from build123d import *

# Parameters (mm, degrees)
SKETCH1_R                       = 4.7625
BOSS_EXTRUDE1_DEPTH             = 6.35
F_14_0_182_DIAMETER_HOLE1_D     = 4.6228
F_14_0_182_DIAMETER_HOLE1_DEPTH = 2.54
F_14_0_182_DIAMETER_HOLE1_TIP   = 1.388829235


with BuildPart() as part:
    # Sketch1 → Boss-Extrude1 (new body)
    with BuildSketch(Plane(origin=(0, 0, 0), x_dir=(1, 0, 0), z_dir=(0, 1, 0))):
        with BuildLine():
            Line((-2.715472603, -50.452570894), (-16.449210706, -36.716165316))
            Line((-16.449210706, -36.716165316), (-7.143929399, -5.302062091))
            ThreePointArc((-7.143929399, -5.302062091), (-4.881213446, -3.126502672), (-1.85461271, -3.95874678))
            Line((-1.85461271, -3.95874678), (13.315573809, -19.128933299))
            Line((13.315573809, -19.128933299), (15.879471691, -10.753687697))
            Line((15.879471691, -10.753687697), (2.2197595, 40.561165667))
            Line((2.2197595, 40.561165667), (-6.994225827, 38.108456959))
            Line((-6.994225827, 38.108456959), (-46.728023778, -55.399752843))
            Line((-46.728023778, -55.399752843), (-12.38156047, -66.157106701))
            ThreePointArc((-12.38156047, -66.157106701), (-1.47172138, -62.045085351), (-2.715472603, -50.452570894))
        make_face()
        with Locations(Location((-9.583361485, -57.052398719, 0), (0, 0, 270))):
            Circle(SKETCH1_R, mode=Mode.SUBTRACT)
    extrude(amount=BOSS_EXTRUDE1_DEPTH)

    # #14 (0.182) Diameter Hole1
    with Locations(Plane(origin=(-19.975553156, 0, 63.778659005), x_dir=(0.9542892760421928, 0, 0.29888455569143674), z_dir=(-0.29888455569143674, 0, 0.9542892760421928))):
        with Locations((-25.620921468, 3.175)):
            Hole(F_14_0_182_DIAMETER_HOLE1_D / 2, depth=F_14_0_182_DIAMETER_HOLE1_DEPTH)
            with Locations((0, 0, -(F_14_0_182_DIAMETER_HOLE1_DEPTH + F_14_0_182_DIAMETER_HOLE1_TIP / 2))):  # 118° drill point
                Cone(0, F_14_0_182_DIAMETER_HOLE1_D / 2, F_14_0_182_DIAMETER_HOLE1_TIP, mode=Mode.SUBTRACT)


solid = part.part
Could you check a few things on this model? Use its own coordinates, in mm. A direction names the side the tool comes from. Coordinates: 2 decimals unless noted, no trailing zeros. Write each loop counter-clockwise with the first axis right and the second up, starting at its lowest first coordinate (ties: lowest second). Pieces come first, ordered by that corner, then holes. Notation, with made-up numbers: (19.25, -39.5) - (68.25, -39.5) arc R31 cw to (68.25, -9.5) - close; hole circle Ø5 at (-4, 79). An arc over 180 degrees is marked (long way). Write item = value, one per line.
1) Suppose I cut it at A-A on z = 7. Please give me the cut outline in (x, y).
Result set:
outline = (-26.16, 0) - (-7.65, 0) - (-7.65, 6.35) - (-26.16, 6.35) - close; (1.19, 0) - (14.88, 0) - (14.88, 6.35) - (1.19, 6.35) - close
2) For faces 1 (the flat face through (-9.486, 3.131, 43.681)), 2 (the cylindrical face through (-4.93, 3.13, 3.14)), 3 (the flat face through (-26.583, 3.131, 7.991)), 4 (the conical face through (-42.958, 3.296, 52.716)), 5 (the flat face through (-16, 6.35, 12)), which set-ups out of +Z, -Z, +X, -X, +Y, -Y let a thin tool reach every point of the face, with its end or its side?
Result set:
face_1 = +X, +Y, -Y
face_2 = +Y, -Y
face_3 = -Z, -X, +Y, -Y
face_4 = none
face_5 = +Z, -Z, +X, -X, +Y
3) Suppose I cut it at C-C on z = 43. Please give me the cut outline in (x, y), plus the area to 3 significant figures.
Result set:
outline = (-41.46, 0) - (-10.17, 0) - (-10.17, 6.35) - (-41.46, 6.35) - close
area = 199 mm2
4) Will these pins go through, and if not, where does the flat tip stop? pin 1 Ø2 at (y, z) = (3, -18.5) entering from -X; pin 2 Ø2 at (y, z) = (3.5, 25.5) entering from +X; pin 3 Ø3 at (x, y) = (-40, 4.5) entering from -Z.
Result set:
pin_1 = -15.75
pin_2 = -12.83
pin_3 = 36.04
5) Please list where these lines run through material, in increasing order: line 1 (X direction, y = 5.75, z = 14); line 2 (X direction, y = 4.5, z = 12); line 3 (Z direction, x = -18, y = 2). Write a range as [from, to].
Result set:
line_1 = [-29.14, -9.72], [8.19, 14.89]
line_2 = [-28.29, -9.13], [6.19, 15.5]
line_3 = [-12.21, 64.4]
6) Suppose I cut it at B-B on x = 1. Please give me the cut outline in (y, z).
Result set:
outline = (0, -40.24) - (6.35, -40.24) - (6.35, 6.81) - (0, 6.81) - close
7) We'd pull the mould along X, two halves only. Please class faces 6 (the flat face through (9.145, 3.131, -14.545)), 7 (the flat face through (-16, 0, 12)), 8 (the flat face through (5.624, 3.131, 11.438)), 9 (the flat face through (-11.86, 3.13, 21.23)): +X half, -X half, draft (parallel to the pull), parting line (faces both ways), or undercut.
Result set:
face_6 = +X half
face_7 = draft
face_8 = undercut
face_9 = undercut
